from build123d import *

# Parameters (mm, degrees)
BOSS_EXTRUDE1_DEPTH     = 100
CUT_EXTRUDE1_REACH      = 124.68
CUT_EXTRUDE1_END_RADIUS = 55.5
SKETCH4_W               = 33
SKETCH4_H               = 40
SKETCH5_W               = 40
SKETCH5_H               = 15
BOSS_EXTRUDE2_DEPTH     = 15
SKETCH6_W               = 40
SKETCH6_H               = 15
CUT_EXTRUDE2_DEPTH      = 10
SKETCH7_W               = 47
SKETCH7_H               = 15
BOSS_EXTRUDE3_DEPTH     = 5
SKETCH8_W               = 47
SKETCH8_H               = 15
BOSS_EXTRUDE4_DEPTH     = 20
CUT_EXTRUDE3_DEPTH      = 140.772135993
BOSS_EXTRUDE5_DEPTH     = 15


with BuildPart() as part:
    # Sketch1 → Boss-Extrude1 (new body)
    with BuildSketch(Plane.XY):
        with BuildLine():
            Line((-10, 54.591666031), (-10, -1.408333969))
            ThreePointArc((-10, -1.408333969), (-7.071067812, -8.479401781), (0, -11.408333969))
            Line((0, -11.408333969), (20, -11.408333969))
            Line((20, -11.408333969), (20, -26.408333969))
            Line((20, -26.408333969), (-20, -26.408333969))
            Line((-20, -26.408333969), (-20, -51.771130952))
            ThreePointArc((-20, -51.771130952), (-55.256322222, 5.195079839), (-10, 54.591666031))
        make_face()
    extrude(amount=BOSS_EXTRUDE1_DEPTH)

    # Cut-Extrude1: up to this cylinder (the profile starts inside it)
    cut_extrude1_end = Plane(origin=(0, 0, 53.5), z_dir=(0, 0, -1)) * Cylinder(CUT_EXTRUDE1_END_RADIUS, 361.36, mode=Mode.PRIVATE)
    # Sketch4 → Cut-Extrude1 (cut, up to the surface)
    with BuildSketch(Plane(origin=(-10, 0, 0), x_dir=(0, 0, -1), z_dir=(1, 0, 0)), mode=Mode.PRIVATE) as cut_extrude1_sk1:
        with Locations((-53.5, 34.591666031)):
            Rectangle(SKETCH4_W, SKETCH4_H)
    cut_extrude1_tool1 = extrude(cut_extrude1_sk1.sketch, amount=-CUT_EXTRUDE1_REACH, mode=Mode.PRIVATE) & cut_extrude1_end
    add(cut_extrude1_tool1.solids().sort_by_distance((-10, 34.591666, 53.5))[0], mode=Mode.SUBTRACT)

    # Sketch5 → Boss-Extrude2 (add, symmetric)
    with BuildSketch(Plane(origin=(-10, 0, 0), x_dir=(0, 0, -1), z_dir=(1, 0, 0))):
        with Locations((-90, 32.091666031)):
            Rectangle(SKETCH5_W, SKETCH5_H)
    extrude(amount=BOSS_EXTRUDE2_DEPTH, both=True)

    # Sketch6 → Cut-Extrude2 (cut)
    with BuildSketch(Plane(origin=(5, 0, 0), x_dir=(0, 0, -1), z_dir=(1, 0, 0))):
        with Locations((-90, 32.091666031)):
            Rectangle(SKETCH6_W, SKETCH6_H)
    extrude(amount=-CUT_EXTRUDE2_DEPTH, mode=Mode.SUBTRACT)

    # Sketch7 → Boss-Extrude3 (add, symmetric)
    with BuildSketch(Plane(origin=(-10, 0, 0), x_dir=(0, 0, -1), z_dir=(1, 0, 0))):
        with Locations((-13.5, 32.091666031)):
            Rectangle(SKETCH7_W, SKETCH7_H)
    extrude(amount=BOSS_EXTRUDE3_DEPTH, both=True)

    # Sketch8 → Boss-Extrude4 (add)
    with BuildSketch(Plane(origin=(-5, 0, 0), x_dir=(0, 0, -1), z_dir=(1, 0, 0))):
        with Locations((-13.5, 32.091666031)):
            Rectangle(SKETCH8_W, SKETCH8_H)
    extrude(amount=-BOSS_EXTRUDE4_DEPTH)

    # Sketch9 → Cut-Extrude3 (cut, through all)
    with BuildSketch(Plane(origin=(0, -11.408333969, 0), x_dir=(1, 0, 0), z_dir=(0, 1, 0))):
        with BuildLine():
            Line((15, -10), (15, -90))
            ThreePointArc((15, -90), (10, -95), (5, -90))
            Line((5, -90), (5, -10))
            ThreePointArc((5, -10), (10, -5), (15, -10))
        make_face()
    extrude(amount=-CUT_EXTRUDE3_DEPTH, mode=Mode.SUBTRACT)

    # Sketch10 → Boss-Extrude5 (add)
    with BuildSketch(Plane.XY.offset(100)):
        with BuildLine():
            Line((20, -26.408333969), (20, -21.408333969))
            Line((20, -21.408333969), (-55.235044142, -5.416631669))
            ThreePointArc((-55.235044142, -5.416631669), (-44.254717417, -33.638955135), (-20, -51.771130952))
            Line((-20, -51.771130952), (-20, -26.408333969))
            Line((-20, -26.408333969), (20, -26.408333969))
        make_face()
    extrude(amount=BOSS_EXTRUDE5_DEPTH)


solid = part.part
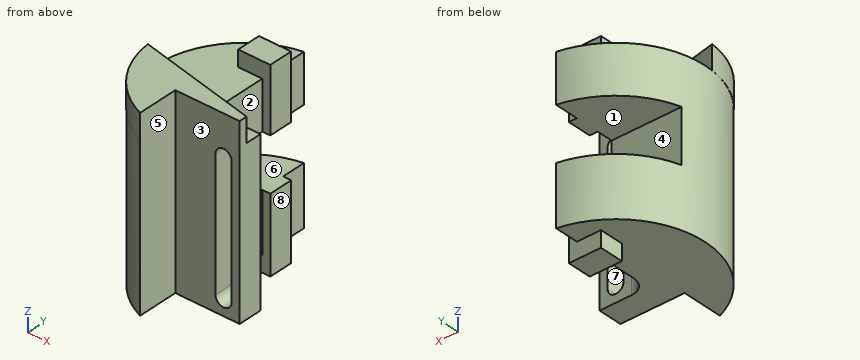
Could you check a few things on this model? Use its own coordinates, in mm. Face numbers are marked on the shaded views. A direction names the side the tool comes from. Give positions to 0.01 mm unless a question says otherwise; leave off trailing zeros. Order: outer loops, then holes, each group sorted by start corner. A loop starts at its lowest first (then second) coordinate and runs counter-clockwise, first axis right, second up. Notation, with made-up numbers: (-37, 13) -> (-30, 13) arc R17 ccw to (-30, 30) -> close; hole circle Ø3 at (6.25, -5.75). An arc over 180 degrees is marked (long way). Answer in a Markdown table with one row per item. Add a question column.
Item 1: I'm going to push flat-ended pins straight in: P1, Ø8, axis at y = -29.5, z = 95.5, coming from the +X side; P2, Ø16.5, axis at x = -11, y = 31.5, coming from the +Z side; P3, Ø10, axis at x = -24.5, z = 46, coming from the +Y side; P4, Ø8, axis at y = 9, z = 54, coming from the +X side. Where does each tip first touch, or does it pass through?
Item 2: Imagine slicing it at D-D (x = -1.5). List the corners of the cut face in (y, z) for me.
Item 3: Please list where these lines run through material, in increasing order: probe 1 along Z at (x, y) = (-22, 24); probe 2 along Y at (x, z) = (-16.5, 64.5); probe 3 along Y at (x, z) = (6.5, 99).
Item 4: Imagine slicing it at A-A (z = 13). List the corners of the cut face in (x, y) for me.
Item 5: For the marked faces 5, 6, 7 and 8, which set-ups out of +Z, -Z, +X, -X, +Y, -Y let a thin tool reach every point of the face, with its end or its side?
Item 6: Imagine slicing it at C-C (x = 10). List the corners of the cut face in (y, z) for me, and give its area (3 significant figures).
Item 7: We'd pull the mould along Y, two halves only. Please class the marked faces 1, 2, 3 and 4: pulls with the +Y half, pulls with the -Y half, needs draft (parallel to the pull), parting line crosses it, or undercut.
Item 8: Imagine slicing it at B-B (y = 43). List the corners of the cut face in (x, z) for me, and give its area (3 significant figures).
Result:
| question | item | result |
|---|---|---|
| 1 | P1 | x = 20 |
| 1 | P2 | z = 110 |
| 1 | P3 | y = 14.59 |
| 1 | P4 | x = -10 |
| 2 | outline | (-26.41, 0) -> (-11.3, 0) -> (-11.3, 100) -> (-16.84, 100) -> (-16.84, 115) -> (-26.41, 115) -> close |
| 3 | probe 1 | 0 to 37, 70 to 100 |
| 3 | probe 2 | -26.41 to 14.59 |
| 3 | probe 3 | -26.41 to -11.41 |
| 4 | outline | (-20, -51.77) -> (-20, -26.41) -> (5, -26.41) -> (5, -11.41) -> (0, -11.41) arc R10 cw to (-10, -1.41) -> (-10, 24.59) -> (-5, 24.59) -> (-5, 39.59) -> (-10, 39.59) -> (-10, 54.59) arc R55.5 ccw to start; (15, -26.41) -> (20, -26.41) -> (20, -11.41) -> (15, -11.41) -> close |
| 5 | face 5 | +Z, -Z, +X, -Y |
| 5 | face 6 | +X, -X, +Y |
| 5 | face 7 | +Y, -Y |
| 5 | face 8 | +Z, -Z, +X, +Y |
| 6 | outline | (-26.41, 0) -> (-11.41, 0) -> (-11.41, 5) -> (-26.41, 5) -> close; (-26.41, 95) -> (-11.41, 95) -> (-11.41, 100) -> (-19.28, 100) -> (-19.28, 115) -> (-26.41, 115) -> close |
| 6 | area | 257 mm2 |
| 7 | face 1 | needs draft |
| 7 | face 2 | undercut |
| 7 | face 3 | pulls with the -Y half |
| 7 | face 4 | pulls with the +Y half |
| 8 | outline | (-35.09, 0) -> (-10, 0) -> (-10, 37) -> (-35.09, 37) -> close; (-35.09, 70) -> (-10, 70) -> (-10, 100) -> (-35.09, 100) -> close |
| 8 | area | 1,680 mm2 |
